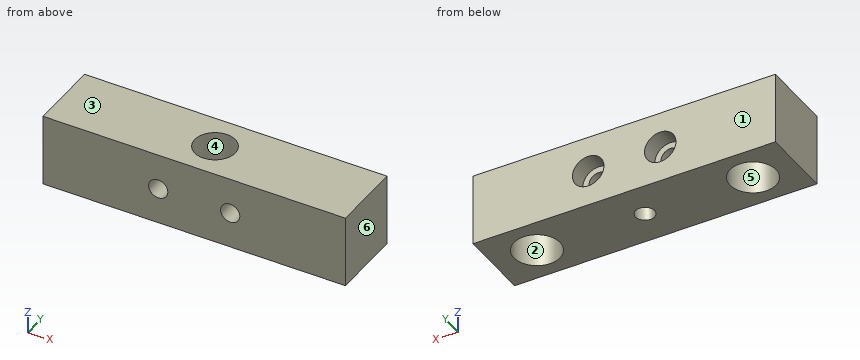
```python
from build123d import *

# Parameters (mm, degrees)
SKETCH1_W                                            = 106.68
SKETCH1_H                                            = 25.4
BOSS_EXTRUDE1_DEPTH                                  = 25.4
SKETCH1_3_R                                          = 8.128
CUT_EXTRUDE1_DEPTH                                   = 19.05
CBORE_FOR_1_4_BINDING_HEAD_MACHINE_SCREW_D           = 6.7564
CBORE_FOR_1_4_BINDING_HEAD_MACHINE_SCREW_CBORE_D     = 14.2875
CBORE_FOR_1_4_BINDING_HEAD_MACHINE_SCREW_CBORE_DEPTH = 19.05
CBORE_FOR_1_4_SOCKET_HEAD_CAP_SCREW1_D               = 6.7564
CBORE_FOR_1_4_SOCKET_HEAD_CAP_SCREW1_CBORE_D         = 11.1125
CBORE_FOR_1_4_SOCKET_HEAD_CAP_SCREW1_CBORE_DEPTH     = 6.35


with BuildPart() as part:
    # Sketch1 → Boss-Extrude1 (new body)
    with BuildSketch(Plane.XY):
        Rectangle(SKETCH1_W, SKETCH1_H)
    extrude(amount=BOSS_EXTRUDE1_DEPTH)

    # Sketch1<3> → Cut-Extrude1 (cut)
    with BuildSketch(Plane.XY):
        with Locations(Location((-38.1, 0, 0), (0, 0, 180))):
            Circle(SKETCH1_3_R)
        with Locations(Location((38.1, 0, 0), (0, 0, 180))):
            Circle(SKETCH1_3_R)
    extrude(amount=CUT_EXTRUDE1_DEPTH, mode=Mode.SUBTRACT)

    # CBORE for 1/4 Binding Head Machine Screw1 (through all)
    with Locations(Plane.XY.offset(25.4)):
        with Locations((0, 0)):
            CounterBoreHole(CBORE_FOR_1_4_BINDING_HEAD_MACHINE_SCREW_D / 2, CBORE_FOR_1_4_BINDING_HEAD_MACHINE_SCREW_CBORE_D / 2, CBORE_FOR_1_4_BINDING_HEAD_MACHINE_SCREW_CBORE_DEPTH)

    # CBORE for 1/4 Socket Head Cap Screw1 (through all)
    with Locations(Plane(origin=(0, 12.7, 0), x_dir=(1, 0, 0), z_dir=(0, 1, 0))):
        with Locations((12.7, -12.7), (-12.7, -12.7)):
            CounterBoreHole(CBORE_FOR_1_4_SOCKET_HEAD_CAP_SCREW1_D / 2, CBORE_FOR_1_4_SOCKET_HEAD_CAP_SCREW1_CBORE_D / 2, CBORE_FOR_1_4_SOCKET_HEAD_CAP_SCREW1_CBORE_DEPTH)


solid = part.part
```
Read the model definition and answer for the solid it produces. Units are mm, in the model's axes. Face numbers are marked on the shaded views. A direction names the side the tool comes from. Round coordinates to 2 decimals unless told otherwise and drop trailing zeros. Write each loop counter-clockwise with the first axis right and the second up, starting at its lowest first coordinate (ties: lowest second). Pieces come first, ordered by that corner, then holes. Notation, with made-up numbers: M 15,-10.75 L 26,-10.75 A15 cw 26,-3.75 Z; hole C 73,-11 d6. An arc over 180 degrees is marked long. One line per item, written item: value.
Q1. Find section B-B on x = 0. Write down the section's boundary in (y, z), plus the area to 3 significant figures.
Data:
outline: M -12.7,0 L -3.38,0 L -3.38,6.35 L -7.14,6.35 L -7.14,25.4 L -12.7,25.4 Z; M 3.38,0 L 12.7,0 L 12.7,25.4 L 7.14,25.4 L 7.14,6.35 L 3.38,6.35 Z
area: 330 mm2
Q2. Find section D-D on y = -10.75. Write down the section's boundary in (x, z).
Data:
outline: M -53.34,0 L 53.34,0 L 53.34,25.4 L -53.34,25.4 Z; hole C -12.7,12.7 d6.76; hole C 12.7,12.7 d6.76
Q3. Find section A-A on y = 0. Write down the section's boundary in (x, z).
Data:
outline: M -53.34,0 L -46.23,0 L -46.23,19.05 L -29.97,19.05 L -29.97,0 L -3.38,0 L -3.38,6.35 L -7.14,6.35 L -7.14,25.4 L -53.34,25.4 Z; M 3.38,0 L 29.97,0 L 29.97,19.05 L 46.23,19.05 L 46.23,0 L 53.34,0 L 53.34,25.4 L 7.14,25.4 L 7.14,6.35 L 3.38,6.35 Z; hole C -12.7,12.7 d6.76; hole C 12.7,12.7 d6.76
Q4. Find section C-C on z = 3.5. Write down the section's boundary in (x, y), plus the area to 3 significant figures.
Data:
outline: M -53.34,-12.7 L 53.34,-12.7 L 53.34,12.7 L -53.34,12.7 Z; hole C -38.1,0 d16.26; hole C 0,0 d6.76; hole C 38.1,0 d16.26
area: 2,260 mm2
Q5. Straight lines are drawn through the part: line 1 (Y direction, x = 37.5, z = 13); line 2 (Z direction, x = -12.7, y = -5.75); line 3 (Y direction, x = 0, z = 18). For each, find the intervals that lie inside material, in ascending order. Write a range as [from, to].
Data:
line 1: [-12.7, -8.11], [8.11, 12.7]
line 2: [0, 9.32], [16.08, 25.4]
line 3: [-12.7, -7.14], [7.14, 12.7]
Q6. Which of the six approach directions +Z, -Z, +X, -X, +Y, -Y give full straight-line access (tool end or side, diameter ignored) to the marked faces 1 and 2?
Data:
face 1: +Z, -Z, +X, -X, +Y
face 2: -Z
Q7. For a pull along X with two mould halves and no side action, classify the marked faces 3, 4, 5 and 6 as +X half, -X half, draft (parallel to the pull), parting line (faces both ways), or undercut.
Data:
face 3: draft
face 4: undercut
face 5: undercut
face 6: +X half
Q8. Flat-ended cylindrical pins translate along their axes: pin 1 Ø8 at (x, y) = (-34.5, 1.5) entering from -Z; pin 2 Ø10 at (x, y) = (24, 0) entering from -Z; pin 3 Ø6 at (x, z) = (-12.7, 12.7) entering from -Y; pin 4 Ø5.5 at (x, z) = (15, 14) entering from +Y. Find the tip coordinate at first contact, or state that the pin passes through.
Data:
pin 1: z = 19.05
pin 2: z = 0
pin 3: through
pin 4: y = 6.35
